Geometry check sheet. Reference: the model listing, model coordinates, mm. A direction names the side the tool comes from. Round coordinates to 2 decimals unless told otherwise and drop trailing zeros. Write each loop counter-clockwise with the first axis right and the second up, starting at its lowest first coordinate (ties: lowest second). Pieces come first, ordered by that corner, then holes.
Item 1: Cross-section at D-D (z = -11). Enter the section's corners in (x, y), then the cut area to 3 significant figures.
Item 2: Cross-section at C-C (y = -85). Enter the section's corners in (x, z).
Item 3: Scan lines: probe 1 along Z at (x, y) = (7, -29.5); probe 2 along Z at (x, y) = (-6.5, -7.5); probe 3 along X at (y, z) = (-10, 81.25). Record each from-to range of solid material in increasing order.
Item 4: Cross-section at B-B (z = 32.5). Enter the section's corners in (x, y), then the cut area to 3 significant figures.
Item 5: Draft check along Z on faces 1 (the face through (10, -47, 71)), 2 (the face through (0, -72, 2)), 3 (the face through (-7, -34, -5)). Enter one of: pulls with the +Z half, pulls with the -Z half, needs draft (parallel to the pull), parting line crosses it, or undercut.
Item 6: Depth check by flat-ended pin: P1, Ø10, axis at x = -5.5, z = -8, coming from the -Y side; P2, Ø2, axis at x = -5.5, z = 15, coming from the +Y side; P3, Ø5, axis at x = 8.5, y = -55, coming from the +Z side; P4, Ø6, axis at x = -6, y = -39.5, coming from the -Z side. Enter the tip coordinate at first touch or a pass-through.
Item 7: Cross-section at A-A (y = -44). Enter the section's corners in (x, z).
Item 8: Access from +Z, -Z, +X, -X, +Y, -Y to the whole of each face (thin tool, end or side, straight path). Record for faces 4 (the face through (-4, -81, 21)), 5 (the face through (-6.96, -75.15, 71.99)), 6 (the face through (-7, -78, 35)).
from build123d import *

# Parameters (mm, degrees)
BOSS_EXTRUDE2_DEPTH              = 4
BOSS_EXTRUDE3_DEPTH              = 10
BOSS_EXTRUDE6_DEPTH              = 25
CUT_EXTRUDE3_DEPTH               = 25
M12X1_5_TAPPED_HOLE1_D           = 10.5
M12X1_5_TAPPED_HOLE1_DEPTH       = 25
M12X1_5_TAPPED_HOLE1_CSINK_D     = 12.05
M12X1_5_TAPPED_HOLE1_CSINK_ANGLE = 90
FILLET1_R                        = 2


with BuildPart() as part:
    # Sketch1 → Boss-Extrude2 (new, symmetric)
    with BuildSketch(Plane(origin=(0, 0, 0), x_dir=(0, 0, -1), z_dir=(1, 0, 0))):
        with BuildLine():
            ThreePointArc((-65, -98), (-86.213203, -89.213203), (-95, -68))
            Line((-95, -68), (-95, 0))
            Line((-95, 0), (-75, 0))
            Line((-75, 0), (-75, -68))
            ThreePointArc((-75, -68), (-72.071068, -75.071068), (-65, -78))
            Line((-65, -78), (-5, -78))
            ThreePointArc((-5, -78), (2.071068, -75.071068), (5, -68))
            Line((5, -68), (5, 0))
            Line((5, 0), (25, -30))
            Line((25, -30), (25, -68))
            ThreePointArc((25, -68), (16.213203, -89.213203), (-5, -98))
            Line((-5, -98), (-65, -98))
        make_face()
    extrude(amount=BOSS_EXTRUDE2_DEPTH, both=True)

    # Sketch1<5> → Boss-Extrude3 (add, symmetric)
    with BuildSketch(Plane(origin=(0, 0, 0), x_dir=(0, 0, -1), z_dir=(1, 0, 0))):
        with BuildLine():
            ThreePointArc((-65, -78), (-72.071068, -75.071068), (-75, -68))
            Line((-75, -68), (-75, 0))
            Line((-75, 0), (-70, 0))
            Line((-70, 0), (-70, -68))
            ThreePointArc((-70, -68), (-68.535534, -71.535534), (-65, -73))
            Line((-65, -73), (-5, -73))
            ThreePointArc((-5, -73), (-1.464466, -71.535534), (0, -68))
            Line((0, -68), (0, 0))
            Line((0, 0), (5, 0))
            Line((5, 0), (5, -68))
            ThreePointArc((5, -68), (2.071068, -75.071068), (-5, -78))
            Line((-5, -78), (-65, -78))
        make_face()
    extrude(amount=BOSS_EXTRUDE3_DEPTH, both=True)

    # Sketch2 → Boss-Extrude6 (add)
    with BuildSketch(Plane.XY.offset(95)):
        with BuildLine():
            Line((-10, -10), (-10, -23))
            Line((-10, -23), (10, -23))
            Line((10, -23), (10, -10))
            ThreePointArc((10, -10), (0, 0), (-10, -10))
        make_face()
    extrude(amount=-BOSS_EXTRUDE6_DEPTH)

    # Sketch4 → Cut-Extrude3 (cut)
    with BuildSketch(Plane.XY.offset(95)):
        with BuildLine():
            Line((10, 0), (4, 0))
            Line((4, 0), (4, -0.834849))
            ThreePointArc((4, -0.834849), (8.3666, -4.522774), (10, -10))
            Line((10, -10), (10, 0))
        make_face()
        with BuildLine():
            Line((-10, 0), (-10, -10))
            ThreePointArc((-10, -10), (-8.3666, -4.522774), (-4, -0.834849))
            Line((-4, -0.834849), (-4, 0))
            Line((-4, 0), (-10, 0))
        make_face()
        with BuildLine():
            Line((-4, 0), (-4, -0.834849))
            ThreePointArc((-4, -0.834849), (-2.043096, -0.210937), (0, 0))
            Line((0, 0), (-4, 0))
        make_face()
        with BuildLine():
            Line((4, 0), (0, 0))
            ThreePointArc((0, 0), (2.043096, -0.210937), (4, -0.834849))
            Line((4, -0.834849), (4, 0))
        make_face()
    extrude(amount=-CUT_EXTRUDE3_DEPTH, mode=Mode.SUBTRACT)

    # M12x1.5 Tapped Hole1
    with Locations(Plane.XY.offset(95)):
        with Locations((0, -10)):
            CounterSinkHole(M12X1_5_TAPPED_HOLE1_D / 2, M12X1_5_TAPPED_HOLE1_CSINK_D / 2, depth=M12X1_5_TAPPED_HOLE1_DEPTH, counter_sink_angle=M12X1_5_TAPPED_HOLE1_CSINK_ANGLE)

    # Fillet1
    fillet1_edges = [part.edges().sort_by_distance(p)[0] for p in [
        (-7, -23, 75),
        (7, -23, 75),
    ]]
    fillet(fillet1_edges, radius=FILLET1_R)


solid = part.part
Resolved:
1. outline: (-4, -93.38) - (4, -93.38) - (4, -9) - (-4, -9) - close
1. area: 675 mm2
2. outline: (-4, -19.72) - (4, -19.72) - (4, 89.72) - (-4, 89.72) - close
3. probe 1: z = -5 to 0, 70 to 75
3. probe 2: z = -5 to 0, 70 to 95
3. probe 3: x = -10 to -5.25, 5.25 to 10
4. outline: (-10, -78) - (-4, -78) - (-4, -98) - (4, -98) - (4, -78) - (10, -78) - (10, -73) - (-10, -73) - close
4. area: 260 mm2
5. face 1: needs draft
5. face 2: undercut
5. face 3: pulls with the -Z half
6. P1: stops at y = -96.85
6. P2: stops at y = -73
6. P3: stops at z = 75
6. P4: stops at z = -25
7. outline: (-10, -5) - (-4, -5) - (-4, -25) - (4, -25) - (4, -5) - (10, -5) - (10, 0) - (-10, 0) - close; (-10, 70) - (10, 70) - (10, 75) - (4, 75) - (4, 95) - (-4, 95) - (-4, 75) - (-10, 75) - close
8. face 4: -X, -Y
8. face 5: +Z, -X, -Y
8. face 6: +Z, -Z, -X, -Y
